Can you work these out from the drawing? Everything is in mm from the part's minimum corner. Round coordinates to 2 decimals unless told otherwise and drop trailing zeros. Write each loop counter-clockwise with the first axis right and the second up, starting at its lowest first coordinate (ties: lowest second). Pieces come first, ordered by that corner, then holes. Notation, with made-up numbers: (24, 5.5) - (33, 5.5) arc R24 cw to (33, 37.5) - close; hole circle Ø4 at (73, -22.5). An arc over 180 degrees is marked (long way). One line per item, written item: value. Start each with the question number.
Item 1: Imagine slicing it at A-A, the plane x = 0.4. Please give me the cut outline in (y, z), then the cut area to 3 significant figures.
Item 2: For P1, Ø1, axis at x = 0.5, y = 3.5, coming from the -Z side; P2, Ø0.6, axis at x = 0.5, y = 38.5, coming from the +Z side; P3, Ø0.6, axis at x = 1, z = 1, coming from the +Y side, each with a flat end and sliding along its axis, tell me the tip position at first contact or that it passes through.
Item 3: If I drill on line 1 (Z direction, x = 0.8, y = 35.5), over which ranges is the centre line in solid material (lowest first)?
Item 4: Imagine slicing it at B-B, the plane y = 3. Please give me the cut outline in (x, z).
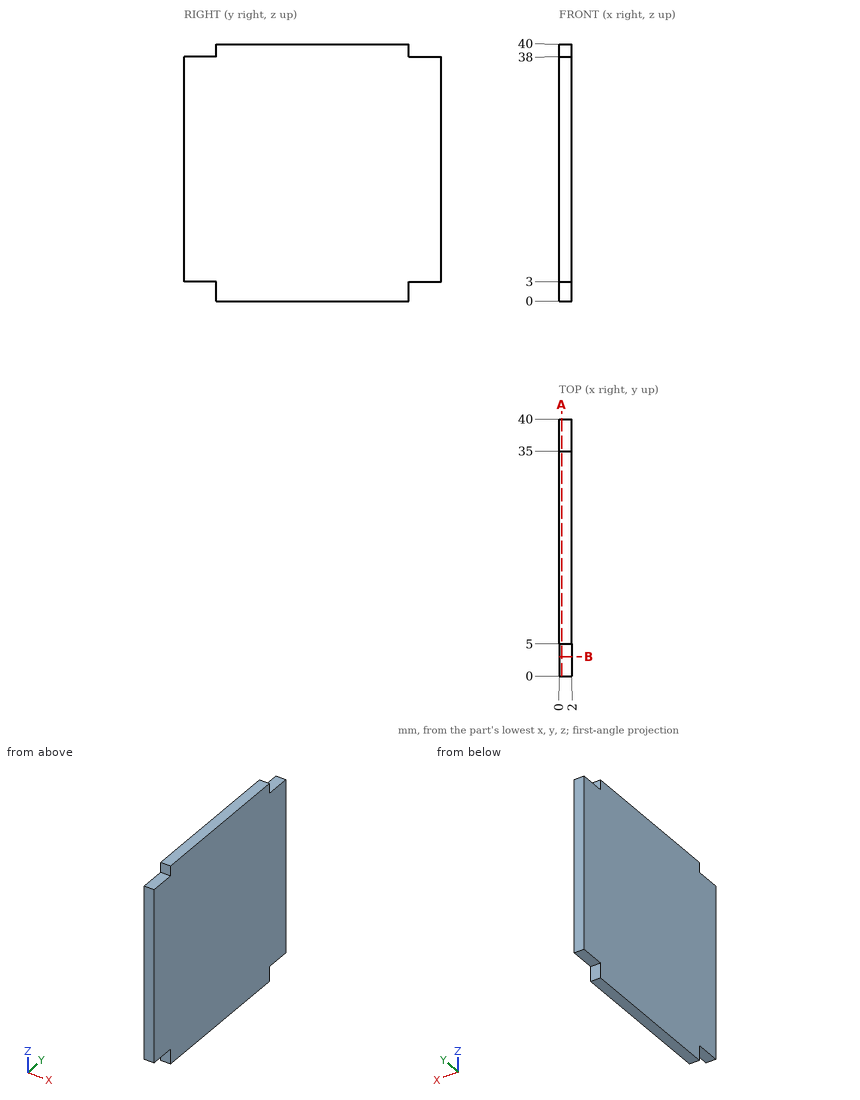
Values follow:
1. outline: (0, 3) - (5, 3) - (5, 0) - (35, 0) - (35, 3) - (40, 3) - (40, 38) - (35, 38) - (35, 40) - (5, 40) - (5, 38) - (0, 38) - close
1. area: 1,550 mm^2
2. P1: stops at z = 3
2. P2: stops at z = 38
2. P3: stops at y = 35
3. line 1: z = 3 to 38
4. outline: (0, 3) - (2, 3) - (2, 38) - (0, 38) - close
